from build123d import *

# Parameters (mm, degrees)
F0_W     = 50.8
F0_H     = 50.8
F1_DEPTH = 50.8
F3_D     = 9.525
F4_D     = 9.525
F6_D     = 9.525
F7_R     = 5.08


# Not quite as in the source:
# - a length typed as a fraction of an inch, garbled in the dataset ("3 / 203.2 mm" for 3/8 in), is restored


with BuildPart() as f1:
    # F0 (on Front) → F1 (new body)
    with BuildSketch(Plane.XZ):
        with Locations((25.4, 25.4)):
            Rectangle(F0_W, F0_H)
    extrude(amount=F1_DEPTH)

    # F3 (through all)
    with Locations(Plane(origin=(0, 0, 0), x_dir=(0, -1, 0), z_dir=(-1, 0, 0))):
        with Locations((12.7, 38.1), (38.1, 38.1), (38.1, 12.7), (12.7, 12.7)):
            Hole(F3_D / 2)

    # F4 (through all)
    with Locations(Plane(origin=(0, 0, 0), x_dir=(1, 0, 0), z_dir=(0, 1, 0))):
        with Locations((38.1, -38.1), (12.7, -38.1), (12.7, -12.7), (38.1, -12.7)):
            Hole(F4_D / 2)

    # F6 (through all)
    with Locations(Plane.XY.offset(50.8)):
        with Locations((12.7, -12.7), (38.1, -12.7), (38.1, -38.1), (12.7, -38.1)):
            Hole(F6_D / 2)

    # F7
    f7_edges = [f1.edges().sort_by_distance(p)[0] for p in [
        (25.4, -50.8, 50.8),
        (0, -25.4, 50.8),
        (50.8, -25.4, 50.8),
        (25.4, 0, 50.8),
        (50.8, 0, 25.4),
        (0, 0, 25.4),
        (25.4, 0, 0),
        (50.8, -25.4, 0),
        (0, -25.4, 0),
        (25.4, -50.8, 0),
        (0, -50.8, 25.4),
        (50.8, -50.8, 25.4),
    ]]
    fillet(f7_edges, radius=F7_R)


solid = f1.part
Geometry: final body of the model. Coordinates: model frame, mm. Coordinates: 2 decimals unless noted, no trailing zeros. Order: outer loops, then holes, each group sorted by start corner. A loop starts at its lowest first (then second) coordinate and runs counter-clockwise, first axis right, second up. Notation, with made-up numbers: M 19,18.25 L 35,18.25 A23 ccw 35,54.25 Z; hole C 2,76.5 d1. An arc over 180 degrees is marked long. One line per question, with ' | ' between items. Start each with the question number.
Item 1: Pin query (flat end, axial travel): pin 1 Ø7.5 at (x, y) = (38.1, -12.7) entering from -Z. Return the tip coordinate at first contact, or that it passes through.
Item 2: Cut plane C-C, the plane x = 12.7. Count the separate pieces of the cut face and the enclosed holes in it, then the cut area to 3 significant figures.
Item 3: Ray query, probe 1 along Y at (x, z) = (32.5, 13); probe 2 along Z at (x, y) = (25, -38); probe 3 along X at (y, z) = (-46, 38.1). Return the intervals inside material, ascending. Write a range as [from, to].
Item 4: Cut plane A-A, the plane y = -27. Return the cut outline in (x, z) (1 decimal), then the cut area to 3 significant figures.
Item 5: Cut plane B-B, the plane x = 25.5. Return the cut outline in (y, z) (1 decimal), then the cut area to 3 significant figures.
Item 6: Draft query along Y for faces 1 (the cylindrical face through (13.73, -25.53, 42.75)), 2 (the cylindrical face through (49.272, -1.449, 25.684)), 3 (the cylindrical face through (42.858, -12.491, 4.601)). Return one class per face: released by +Y, released by -Y, zero draft, split by the parting line, or undercut.
A:
1) pin 1: passes through
2) separate pieces: 9 | enclosed holes: 0 | area: 986 mm2
3) probe 1: y = [-50.8, -42.85], [-33.35, -17.45], [-7.95, 0] | probe 2: z = [0, 7.94], [17.46, 33.34], [42.86, 50.8] | probe 3: x = [0.01, 7.94], [17.46, 33.34], [42.86, 50.79]
4) outline: M 0,5.1 A5.1 ccw 5.1,0 L 45.7,0 A5.1 ccw 50.8,5.1 L 50.8,45.7 A5.1 ccw 45.7,50.8 L 5.1,50.8 A5.1 ccw 0,45.7 Z; hole C 12.7,12.7 d9.5; hole C 12.7,38.1 d9.5; hole C 38.1,12.7 d9.5; hole C 38.1,38.1 d9.5 | area: 2,270 mm2
5) outline: M -50.8,5.1 A5.1 ccw -45.7,0 L -5.1,0 A5.1 ccw 0,5.1 L 0,45.7 A5.1 ccw -5.1,50.8 L -45.7,50.8 A5.1 ccw -50.8,45.7 Z; hole C -38.1,12.7 d9.5; hole C -38.1,38.1 d9.5; hole C -12.7,12.7 d9.5; hole C -12.7,38.1 d9.5 | area: 2,270 mm2
6) face 1: zero draft | face 2: released by +Y | face 3: undercut
